Could you check a few things on this drawing? It's one solid part, dimensions in mm from its lowest x, y, z. A direction names the side the tool comes from. Coordinates: 2 decimals unless noted, no trailing zeros. Order: outer loops, then holes, each group sorted by start corner. A loop starts at its lowest first (then second) coordinate and runs counter-clockwise, first axis right, second up.
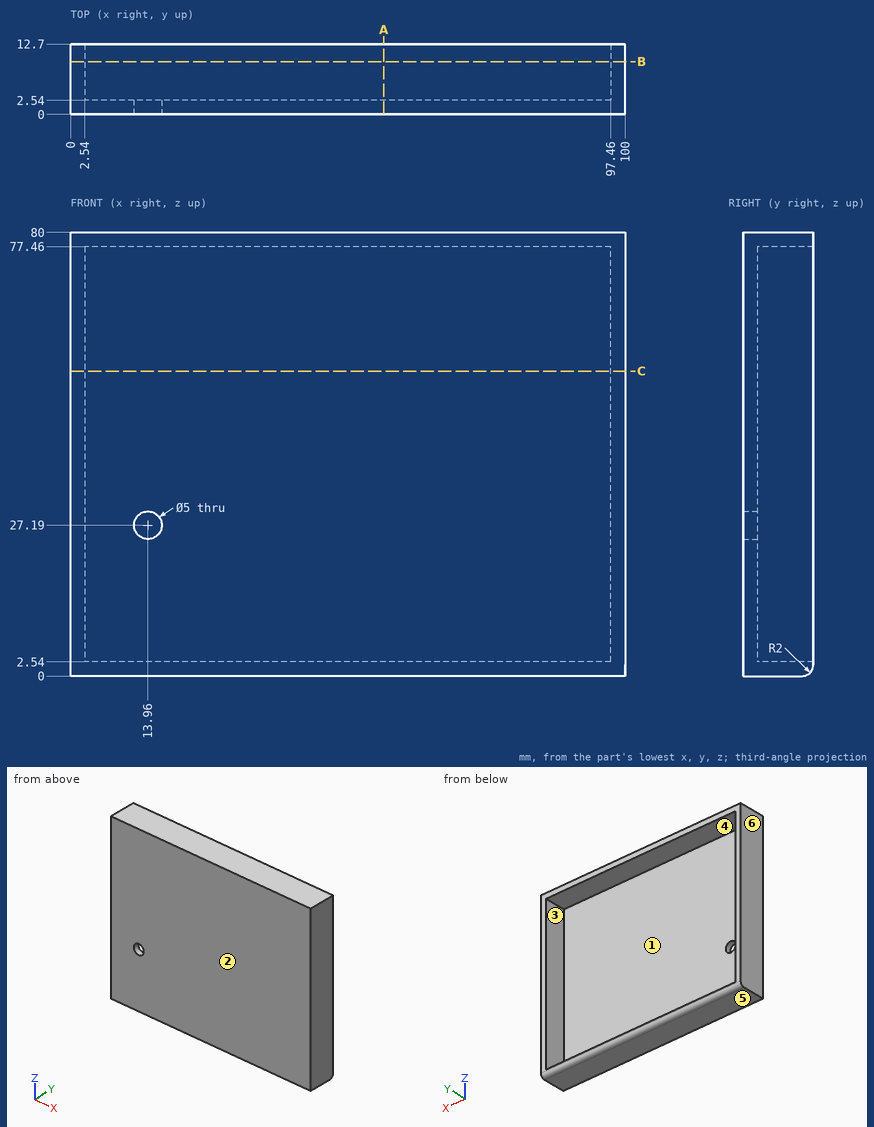
Q1. We'd pull the mould along Z, two halves only. Please class the marked faces 3, 4, 5 and 6: pulls with the +Z half, pulls with the -Z half, needs draft (parallel to the pull), parting line crosses it, or undercut.
Q2. If we section it at A-A on x = 56.5: Write out the boundary of the cut face in (y, z).
Q3. For the marked faces 1 and 2, which set-ups out of +Z, -Z, +X, -X, +Y, -Y let a thin tool reach every point of the face, with its end or its side?
Q4. If we section it at B-B on y = 9.5: Write out the boundary of the cut face in (x, z).
Q5. I need wall thicknesses on L1, parallel to X at y = 3.25, z = 22.5; L2, parallel to Z at x = 60, y = 5.75; L3, parallel to Y at x = 74, z = 48.5. Which ranges of each line are inside material? Lowest first, please.
Q6. If we section it at C-C on z = 55: Write out the boundary of the cut face in (x, y).
Q7. Will this pin go through, and if not, where does the flat tip stop? pin 1 (1.5 mm diameter, centred on x = 25, z = 14.5, fed in from +Y).
Reply:
1. face 3: undercut
1. face 4: undercut
1. face 5: pulls with the -Z half
1. face 6: needs draft
2. outline: (0, 0) - (10.7, 0) arc R2 ccw to (12.7, 2) - (12.7, 2.54) - (2.54, 2.54) - (2.54, 77.46) - (12.7, 77.46) - (12.7, 80) - (0, 80) - close
3. face 1: +Y
3. face 2: +Z, -Z, +X, -X, -Y
4. outline: (0, 0) - (100, 0) - (100, 80) - (0, 80) - close; hole (2.54, 2.54) - (97.46, 2.54) - (97.46, 77.46) - (2.54, 77.46) - close
5. L1: x = 0 to 2.54, 97.46 to 100
5. L2: z = 0 to 2.54, 77.46 to 80
5. L3: y = 0 to 2.54
6. outline: (0, 0) - (100, 0) - (100, 12.7) - (97.46, 12.7) - (97.46, 2.54) - (2.54, 2.54) - (2.54, 12.7) - (0, 12.7) - close
7. pin 1: stops at y = 2.54
